The figure shows three views and two pictorial views of one solid part (mm, origin at its lowest corner). Answer the questions. Round coordinates to 2 decimals unless told otherwise and drop trailing zeros. Write each loop counter-clockwise with the first axis right and the second up, starting at its lowest first coordinate (ties: lowest second). Pieces come first, ordered by that corner, then holes. Notation, with made-up numbers: M 25.5,55 L 58.5,55 A11 cw 58.5,72 Z; hole C 87,-29 d7. An arc over 180 degrees is marked long. Use one line per item in the form item = value. Start each with the question number.
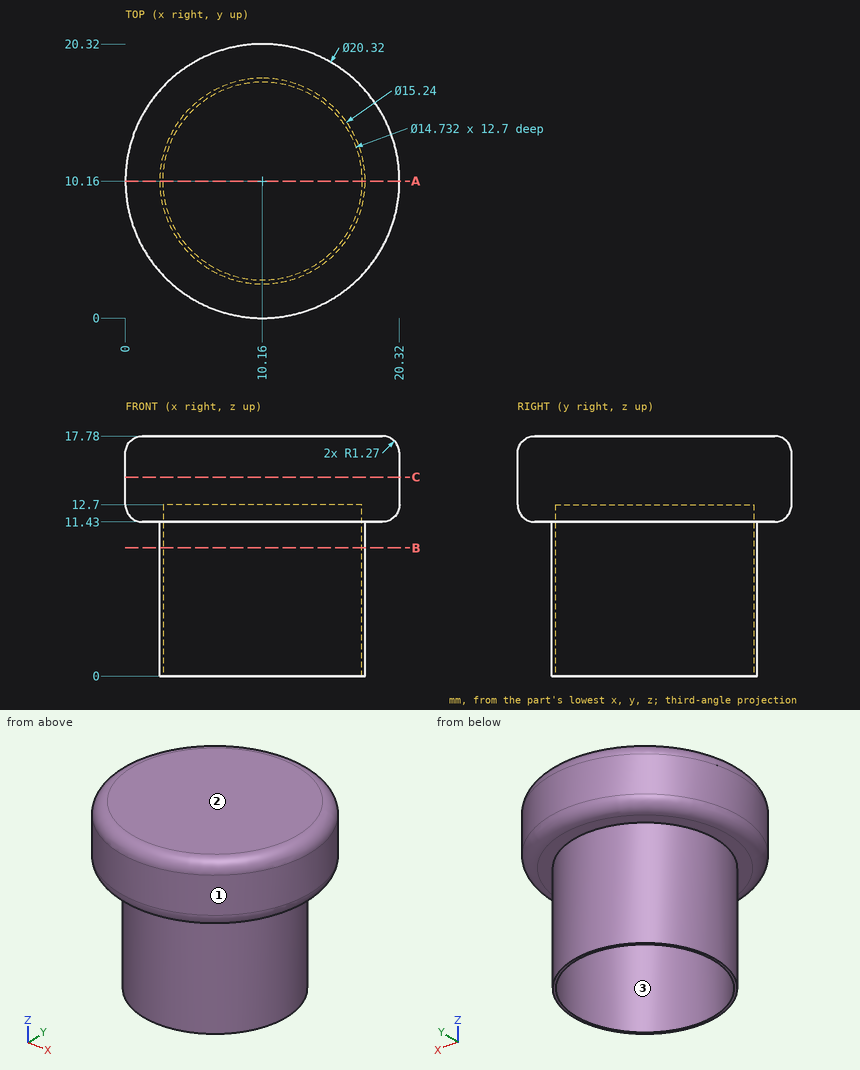
Q1. Find section C-C on z = 14.75. Write down the section's boundary in (x, y), and give its area (3 significant figures).
Q2. For a pull along Y with two mould halves and no side action, classify the marked faces 1, 2 and 3 as +Y half, -Y half, draft (parallel to the pull), parting line (faces both ways), or undercut.
Q3. Each of these flat-tipped pins is pushed along its axis until it touches: pin 1 Ø4.5 at (x, y) = (8.5, 12) entering from -Z; pin 2 Ø1.5 at (y, z) = (13, 12.5) entering from +X; pin 3 Ø8 at (y, z) = (10, 7) entering from -X. Where does it stop, or does it pass through?
Q4. Find section A-A on y = 10.16. Write down the section's boundary in (x, z), and give its area (3 significant figures).
Q5. Straight lines are drawn through the part: line 1 (X direction, y = 10.16, z = 9.75); line 2 (Z direction, x = 5.25, y = 13.5); line 3 (Y direction, x = 9.5, z = 2.5). For each, find the intervals that lie inside material, in ascending order. Write a range as [from, to].
Q6. Find section B-B on z = 9.5. Write down the section's boundary in (x, y), and give its area (3 significant figures).
Response:
q1.outline = C 10.16,10.16 d20.32
q1.area = 324 mm²
q2.face_1 = parting line
q2.face_2 = draft
q2.face_3 = undercut
q3.pin_1 = 12.7
q3.pin_2 = 20.1
q3.pin_3 = 2.54
q4.outline = M 0,12.7 A1.27 ccw 1.27,11.43 L 2.54,11.43 L 2.54,0 L 2.79,0 L 2.79,12.7 L 17.53,12.7 L 17.53,0 L 17.78,0 L 17.78,11.43 L 19.05,11.43 A1.27 ccw 20.32,12.7 L 20.32,16.51 A1.27 ccw 19.05,17.78 L 1.27,17.78 A1.27 ccw 0,16.51 Z
q4.area = 115 mm²
q5.line_1 = [2.54, 2.79], [17.53, 17.78]
q5.line_2 = [12.7, 17.78]
q5.line_3 = [2.57, 2.82], [17.5, 17.75]
q6.outline = C 10.16,10.16 d15.24; hole C 10.16,10.16 d14.73
q6.area = 12.0 mm²
